Geometry check sheet. Reference: the model listing, model coordinates, mm. A direction names the side the tool comes from. Give positions to 0.01 mm unless a question says otherwise; leave off trailing zeros. Write each loop counter-clockwise with the first axis right and the second up, starting at its lowest first coordinate (ties: lowest second). Pieces come first, ordered by that corner, then holes. Notation, with made-up numbers: M 73.5,66 L 125.5,66 A21 cw 125.5,71 Z; hole C 54,-33.5 d1. An arc over 180 degrees is marked long. Write each question's results on one line, items separated by ' | '.
```python
from build123d import *

# Parameters (mm, degrees)
F0_R     = 15
F0_R_2   = 12.5
F1_DEPTH = 20
F4_DEPTH = 2
F5_W     = 34
F5_H     = 34
F6_DEPTH = 2


with BuildPart() as f1:
    # F0 (on Top) → F1 (new body)
    with BuildSketch(Plane.XY):
        Circle(F0_R)
        Circle(F0_R_2, mode=Mode.SUBTRACT)
    extrude(amount=F1_DEPTH)

    # F3 (on offset) → F4 (join)
    with BuildSketch(Plane.XY.offset(8)):
        with BuildLine():
            ThreePointArc((1.396739, 2.073432), (0, -2.5), (-1.396739, 2.073432))
            Line((-1.396739, 2.073432), (-4.714967, 11.576661))
            ThreePointArc((-4.714967, 11.576661), (0, -12.5), (4.714967, 11.576661))
            Line((4.714967, 11.576661), (1.396739, 2.073432))
        make_face()
    extrude(amount=-F4_DEPTH)

    # F5 (on Top) → F6 (join)
    with BuildSketch(Plane.XY):
        with Locations((0.530663, 0)):
            Rectangle(F5_W, F5_H)
    extrude(amount=-F6_DEPTH)


solid = f1.part
```
Q1. Material ranges on probe 1 along Z at (x, y) = (-6, -7); probe 2 along Y at (x, z) = (0, 6.95); probe 3 along Y at (x, z) = (-0.5, 5), recorded low to high. Write a range as [from, to].
Answer key:
probe 1: z = [-2, 0], [6, 8] | probe 2: y = [-15, -2.5], [12.5, 15] | probe 3: y = [-14.99, -12.49], [12.49, 14.99]
Q2. Access from +Z, -Z, +X, -X, +Y, -Y to the whole of each face (thin tool, end or side, straight path). Record for faces 4 (the face through (15.4, 0.2, 0)), 5 (the face through (-16.469, 0, -1)), 6 (the face through (0, 0, 0)).
Answer key:
face 4: +Z | face 5: +Z, -Z, -X, +Y, -Y | face 6: none
Q3. Depth check by flat-ended pin: P1, Ø6, axis at x = -4, z = 16, coming from the -Y side; P2, Ø19.5, axis at x = -0.5, y = -5, coming from the +Z side; P3, Ø10, axis at y = -12.5, z = 17, coming from the +X side; P4, Ø10, axis at x = -5, y = 3, coming from the +Z side. Enter the tip coordinate at first touch or a pass-through.
Answer key:
P1: stops at y = -14.97 | P2: stops at z = 20 | P3: stops at x = 12.99 | P4: stops at z = 8
Q4. Section check A-A (z = 7.25). Enter the section's corners in (x, y), then the cut area to 3 significant figures.
Answer key:
outline: C 0,0 d30; hole M -4.71,11.58 L -1.4,2.07 A2.5 ccw long 1.4,2.07 L 4.71,11.58 A12.5 ccw Z | area: 624 mm2
Q5. Section check D-D (x = 0). Enter the section's corners in (y, z).
Answer key:
outline: M -17,-2 L 17,-2 L 17,0 L 15,0 L 15,20 L 12.5,20 L 12.5,0 L -12.5,0 L -12.5,6 L -2.5,6 L -2.5,8 L -12.5,8 L -12.5,20 L -15,20 L -15,0 L -17,0 Z
Q6. Section check C-C (y = -14). Enter the section's corners in (x, z), then the cut area to 3 significant figures.
Answer key:
outline: M -16.47,-2 L 17.53,-2 L 17.53,0 L 5.39,0 L 5.39,20 L -5.39,20 L -5.39,0 L -16.47,0 Z | area: 283 mm2
Q7. Release check for a two-part mould opening along Y. For faces 1 (the face through (17.531, 0, -1)), 2 (the face through (-14.985, 0.66, 9.86)), 3 (the face through (3.08, 6.89, 7.01)) record: released by +Y, released by -Y, zero draft, split by the parting line, or undercut.
Answer key:
face 1: zero draft | face 2: split by the parting line | face 3: undercut
Q8. Section check B-B (x = 11). Enter the section's corners in (y, z).
Answer key:
outline: M -17,-2 L 17,-2 L 17,0 L 10.2,0 L 10.2,20 L 5.94,20 L 5.94,8 L -5.94,8 L -5.94,20 L -10.2,20 L -10.2,0 L -17,0 Z; hole M -5.94,0 L 5.94,0 L 5.94,6 L -5.94,6 Z
